```python
from build123d import *

# Parameters (mm, degrees)
BOSS_EXTRUDE1_DEPTH      = 40
SKETCH2_R                = 10.076891008
BOSS_EXTRUDE2_DEPTH      = 20
BOSS_EXTRUDE2_DEPTH_BACK = 100
SKETCH5_R                = 10.076891008
CUT_EXTRUDE1_DEPTH       = 101


with BuildPart() as part:
    # Sketch1 → Boss-Extrude1 (new body, symmetric)
    with BuildSketch(Plane.XY):
        with BuildLine():
            Line((0, 50.000244442), (0, 0))
            ThreePointArc((0, 0), (23.127866372, -23.127866372), (46.255732744, 0))
            Line((46.255732744, 0), (46.255732744, 50.000244442))
            Line((46.255732744, 50.000244442), (59.912187173, 50.000244442))
            Line((59.912187173, 50.000244442), (59.912187173, 0))
            ThreePointArc((59.912187173, 0), (22.46707019, -37.445116983), (-14.978046793, 0))
            Line((-14.978046793, 0), (-14.978046793, 50.000244442))
            Line((-14.978046793, 50.000244442), (0, 50.000244442))
        make_face()
    extrude(amount=BOSS_EXTRUDE1_DEPTH, both=True)

    # Sketch2 → Boss-Extrude2 (add, two sides)
    with BuildSketch(Plane.ZY.offset(14.978046793)) as boss_extrude2_sk:
        with BuildLine():
            Line((-23.095980377, -26.1078298), (23.095980377, -26.1078298))
            Line((23.095980377, -26.1078298), (23.095980377, 26.1078298))
            ThreePointArc((23.095980377, 26.1078298), (0, 49.203810178), (-23.095980377, 26.1078298))
            Line((-23.095980377, 26.1078298), (-23.095980377, -26.1078298))
        make_face()
        with Locations((0, 26.1078298)):
            Circle(SKETCH2_R, mode=Mode.SUBTRACT)
    extrude(amount=BOSS_EXTRUDE2_DEPTH)
    extrude(boss_extrude2_sk.sketch, amount=-BOSS_EXTRUDE2_DEPTH_BACK)

    # Sketch5 → Cut-Extrude1 (cut, through all)
    with BuildSketch(Plane.ZY.offset(14.978046793)):
        with Locations((0, 26.1078298)):
            Circle(SKETCH5_R)
    extrude(amount=-CUT_EXTRUDE1_DEPTH, mode=Mode.SUBTRACT)


solid = part.part
```
Here's how the part is built. I have some questions about the finished solid (model axes, mm). A direction names the side the tool comes from. Coordinates: 2 decimals unless noted, no trailing zeros. Order: outer loops, then holes, each group sorted by start corner. A loop starts at its lowest first (then second) coordinate and runs counter-clockwise, first axis right, second up. Notation, with made-up numbers: M 89,72 L 147,72 A16 cw 147,82 Z; hole C 71.5,75 d7. An arc over 180 degrees is marked long. Answer as a JSON object with one key per item and string values. Group by question number.
(1) Suppose I cut it at D-D, the plane y = 4. Please give me the cut outline in (x, z), then the cut area to 3 significant figures.
(2) Suppose I cut it at A-A, the plane y = 34. Please give me the cut outline in (x, z), then the cut area to 3 significant figures.
(3) Suppose I cut it at C-C, the plane x = 39. Please give me the cut outline in (y, z), then the cut area to 3 significant figures.
(4) If we mould it in two halves opening along X, with no side actions, what happens to faces 1 (the face through (59.912, 48, 9)), 2 (the face through (71, 0, 23.096)), 3 (the face through (22.619, -23.122, 31.666))? For each: released by +X, released by -X, zero draft, split by the parting line, or undercut.
(5) I need wall thicknesses on probe 1 along X at (y, z) = (41.5, 27.5); probe 2 along Y at (x, z) = (56.5, 0); probe 3 along Y at (x, z) = (70.5, 0). Which ranges of each line are inside material? Lowest first, please.
(6) For pin 1 (9 mm diameter, centred on x = -26, z = -3.5, fed in from -Y); pin 2 (18 mm diameter, centred on x = 75, y = 0, fed in from -Z); pin 3 (6 mm diameter, centred on x = 5.5, z = 0.5, fed in from -Y), each with a flat end and sliding along its axis, tell me the tip position at first contact or that it passes through.
(7) Suppose I cut it at B-B, the plane z = 0. Please give me the cut outline in (x, y).
(8) Which directions (+Z, -Z, +X, -X, +Y, -Y) give clear straight access to the entire face, cutting with the end or side of a thin tool? Please do faces 4 (the face through (23, 2, -23.096)), 5 (the face through (46.256, 41, 18)), 6 (the face through (23, 1, 23.096)), 7 (the face through (-24.8, 49.2, 0.5)).
Values found:
{
 "1": {"outline": "M -34.98,-23.1 L -14.98,-23.1 L -14.98,-40 L 0,-40 L 0,-23.1 L 46.26,-23.1 L 46.26,-40 L 59.91,-40 L 59.91,-23.1 L 85.02,-23.1 L 85.02,23.1 L 59.91,23.1 L 59.91,40 L 46.26,40 L 46.26,23.1 L 0,23.1 L 0,40 L -14.98,40 L -14.98,23.1 L -34.98,23.1 Z", "area": "6,510 mm^2"},
 "2": {"outline": "M -34.98,-21.71 L -14.98,-21.71 L -14.98,-40 L 0,-40 L 0,-21.71 L 46.26,-21.71 L 46.26,-40 L 59.91,-40 L 59.91,-21.71 L 85.02,-21.71 L 85.02,-6.27 L -34.98,-6.27 Z; M -34.98,6.27 L 85.02,6.27 L 85.02,21.71 L 59.91,21.71 L 59.91,40 L 46.26,40 L 46.26,21.71 L 0,21.71 L 0,40 L -14.98,40 L -14.98,21.71 L -34.98,21.71 Z", "area": "4,750 mm^2"},
 "3": {"outline": "M -33.6,-40 L -16.82,-40 L -16.82,-23.1 L 26.11,-23.1 A23.1 ccw 26.11,23.1 L -16.82,23.1 L -16.82,40 L -33.6,40 Z; hole C 26.11,0 d20.15", "area": "3,840 mm^2"},
 "4": {"face 1": "released by +X", "face 2": "zero draft", "face 3": "undercut"},
 "5": {"probe 1": "x = -14.98 to 0, 46.26 to 59.91", "probe 2": "y = -26.11 to 16.03, 36.18 to 50", "probe 3": "y = -26.11 to 16.03, 36.18 to 49.2"},
 "6": {"pin 1": "stops at y = -26.11", "pin 2": "stops at z = -23.1", "pin 3": "stops at y = -34.74"},
 "7": {"outline": "M -34.98,-26.11 L -4.38,-26.11 A37.45 ccw 49.31,-26.11 L 85.02,-26.11 L 85.02,16.03 L -34.98,16.03 Z; M -34.98,36.18 L 85.02,36.18 L 85.02,49.2 L 59.91,49.2 L 59.91,50 L 46.26,50 L 46.26,49.2 L 0,49.2 L 0,50 L -14.98,50 L -14.98,49.2 L -34.98,49.2 Z"},
 "8": {"face 4": "-Z, +Y", "face 5": "+Y", "face 6": "+Z, +Y", "face 7": "-X, +Y"}
}
